For this review, take the finished solid that the model builds, in its own axes (mm). A direction names the side the tool comes from. Give positions to 0.01 mm unless a question says otherwise; leave off trailing zeros. Write each loop counter-clockwise with the first axis right and the second up, starting at its lowest first coordinate (ties: lowest second). Pieces come first, ordered by that corner, then holes. Notation, with made-up numbers: (53, 53) -> (63, 53) arc R16 ccw to (63, 62) -> close; hole circle Ø2 at (-11, 87.5). An arc over 180 degrees is marked (long way). Return JSON: item names as keys, results as strings.
from build123d import *

# Parameters (mm, degrees)
F3_D     = 6.35
F4_W     = 60.513176
F4_H     = 134.324468
F4_R     = 3.175
F5_DEPTH = 65.258862


with BuildPart() as f1:
    # F0 (on Front) → F1 (revolve)
    with BuildSketch(Plane.XZ):
        Polygon((-7.151507, 0), (23.463517, 0), (23.463517, 65.257862), (-86.5217, 65.257862), (-86.5217, 0), align=None)
    revolve(axis=Axis((-86.5217, 0, 32.628931), (0, 0, 1)))

    # F3 (through all)
    with Locations(Plane(origin=(0, 0, 0), x_dir=(1, 0, 0), z_dir=(0, 0, -1))):
        with Locations((-90.931758, 0)):
            Hole(F3_D / 2)

    # F4 (on face) → F5 (cut, through all)
    with BuildSketch(Plane.XY.offset(65.257862)):
        with Locations((-87.257598, -0.581134)):
            Rectangle(F4_W, F4_H)
        with Locations((-90.931758, 0)):
            Circle(F4_R, mode=Mode.SUBTRACT)
    extrude(amount=-F5_DEPTH, mode=Mode.SUBTRACT)


solid = f1.part
1. Add section A-A, the plane y = 0. State the section outline as (x, z) points, plus the area to 3 significant figures.
Results found:
{"outline": "(-196.51, 0) -> (-117.51, 0) -> (-117.51, 65.26) -> (-196.51, 65.26) -> close; (-57, 0) -> (23.46, 0) -> (23.46, 65.26) -> (-57, 65.26) -> close", "area": "10,400 mm²"}
2. For pin 1 (8 mm diameter, centred on y = -62.5, z = 13, fed in from -X); pin 2 (5 mm diameter, centred on x = -125.5, z = 15, fed in from -Y); pin 3 (6 mm diameter, centred on y = -35.5, z = 34, fed in from -X), all flat-tipped, find the tip position at first contact; note any pin that passes through.
Results found:
{"pin 1": "stops at x = -179.66", "pin 2": "stops at y = -103.76", "pin 3": "stops at x = -191.6"}
3. To check wall thickness, follow probe 1 along Y at (x, z) = (-94.5, 56.5); probe 2 along X at (y, z) = (-51, 55.5); probe 3 along Y at (x, z) = (-75, 6). State the ranges of each line that lie inside material, in increasing order.
Results found:
{"probe 1": "y = -109.7 to -67.74, 66.58 to 109.7", "probe 2": "x = -183.97 to -117.51, -57 to 10.92", "probe 3": "y = -109.38 to -67.74, 66.58 to 109.38"}
4. The part is to be moulded in two halves that separate along Y. For faces 3 (the cylindrical face through (-196.4, 4.84, 33.09)), 4 (the flat face through (-57.001, -2, 33)), 5 (the flat face through (-134, 2, 0)), say which applies: +Y half, -Y half, draft (parallel to the pull), parting line (faces both ways), or undercut.
Results found:
{"face 3": "parting line", "face 4": "undercut", "face 5": "draft"}
5. For faces 1 (the flat face through (-88, 66.581, 33)), 2 (the flat face through (-39, 2, 65.258)), list the 3-axis set-ups (+Z, -Z, +X, -X, +Y, -Y) from which the entire face can be reached by the end or side of a thin tool; tool diameter is ignored.
Results found:
{"face 1": "+Z, -Z", "face 2": "+Z, +X, -X, +Y, -Y"}
6. Add section C-C, the plane z = 47. State the section outline as (x, y) points.
Results found:
{"outline": "circle Ø219.97 at (-86.52, 0); hole (-117.51, -67.74) -> (-57, -67.74) -> (-57, 66.58) -> (-117.51, 66.58) -> close"}
7. Add section D-D, the plane x = -43. State the section outline as (y, z) points.
Results found:
{"outline": "(-101.01, 0) -> (101.01, 0) -> (101.01, 65.26) -> (-101.01, 65.26) -> close"}
8. Add section B-B, the plane x = -104. State the section outline as (y, z) points, plus the area to 3 significant figures.
Results found:
{"outline": "(-108.59, 0) -> (-67.74, 0) -> (-67.74, 65.26) -> (-108.59, 65.26) -> close; (66.58, 0) -> (108.59, 0) -> (108.59, 65.26) -> (66.58, 65.26) -> close", "area": "5,410 mm²"}
